Here's how the part is built. I have some questions about the finished solid (model axes, mm). A direction names the side the tool comes from. Coordinates: 2 decimals unless noted, no trailing zeros. Write each loop counter-clockwise with the first axis right and the second up, starting at its lowest first coordinate (ties: lowest second). Pieces come first, ordered by that corner, then holes. Notation, with made-up numbers: (-31, 13.25) -> (9, 13.25) arc R14 cw to (9, 35.25) -> close; hole circle Ø3 at (66.5, 67). An arc over 180 degrees is marked (long way). Use a Markdown table: item, result. Add a question column.
Item 1: If we mould it in two halves opening along X, with no side actions, what happens to faces 1 (the cylindrical face through (-59.462, -45.594, 6.261)), 2 (the cylindrical face through (184.06, 22.89, 117.82)), 3 (the cylindrical face through (-60.47, -46.367, 6.261))? For each: pulls with the +X half, pulls with the -X half, needs draft (parallel to the pull), parting line crosses it, or undercut.
Item 2: Imagine slicing it at A-A, the plane y = 0. Write out the boundary of the cut face in (x, z), and give its area (3 significant figures).
Item 3: Imagine slicing it at B-B, the plane y = -37. Write out the boundary of the cut face in (x, z).
Item 4: Will these pins go through, and if not, where does the flat tip stop? pin 1 Ø1.5 at (y, z) = (-53.5, 62) entering from -X; pin 2 Ø4 at (y, z) = (34.5, 58) entering from +X; pin 3 Ø3 at (x, y) = (107, -24) entering from +Z.
Item 5: If I drill on line 1 along Z through (x, y) = (179, 2); line 2 along Y through (x, z) = (186.25, 190.5); line 3 along Y through (x, z) = (-43, 60), over which ranges is the centre line in solid material (lowest first)? Write a range as from..to.
Item 6: On a 3-axis mill with a long thin cutter (end or side, diameter ignored), from which of +Z, -Z, +X, -X, +Y, -Y can I reach the whole of each face in a straight line? I mean faces 4 (the cylindrical face through (184.061, -28.699, 121.284)), 5 (the flat face through (190.5, -50, 134)). Say none if no direction works.
```python
from build123d import *

# Parameters (mm, degrees)
F0_R     = 76.2
F0_R_2   = 74.93
F1_DEPTH = 12.7
F2_R     = 76.2
F2_R_2   = 74.93
F3_ANGLE = 90
F4_DEPTH = 12.7


with BuildPart() as f1:
    # F0 (on Top) → F1 (new body)
    with BuildSketch(Plane.XY):
        Circle(F0_R)
        Circle(F0_R_2, mode=Mode.SUBTRACT)
    extrude(amount=F1_DEPTH)

    # F2 (on face) → F3 (revolve)
    with BuildSketch(Plane.XY.offset(12.7)):
        Circle(F2_R)
        Circle(F2_R_2, mode=Mode.SUBTRACT)
    revolve(axis=Axis((177.8, -2.9342612252, 12.7), (0, 1, 0)), revolution_arc=F3_ANGLE)

    # F4 (add): a face of the model
    f4_faces = [f1.faces().sort_by_distance(p)[0] for p in [
        (177.8, 0, 266.4844738531),
    ]]
    extrude(f4_faces, amount=F4_DEPTH)


solid = f1.part
```
Ans:
| question | item | result |
|---|---|---|
| 1 | face 1 | undercut |
| 1 | face 2 | needs draft |
| 1 | face 3 | parting line crosses it |
| 2 | outline | (-76.2, 0) -> (-74.93, 0) -> (-74.93, 12.7) arc R252.73 cw to (177.8, 265.43) -> (190.5, 265.43) -> (190.5, 266.7) -> (177.8, 266.7) arc R254 ccw to (-76.2, 12.7) -> close; (74.93, 0) -> (76.2, 0) -> (76.2, 12.7) arc R101.6 cw to (177.8, 114.3) -> (190.5, 114.3) -> (190.5, 115.57) -> (177.8, 115.57) arc R102.87 ccw to (74.93, 12.7) -> close |
| 2 | area | 774 mm^2 |
| 3 | outline | (-66.61, 0) -> (-65.16, 0) -> (-65.16, 12.7) arc R242.96 cw to (177.8, 255.66) -> (190.5, 255.66) -> (190.5, 257.11) -> (177.8, 257.11) arc R244.41 ccw to (-66.61, 12.7) -> close; (65.16, 0) -> (66.61, 0) -> (66.61, 12.7) arc R111.19 cw to (177.8, 123.89) -> (190.5, 123.89) -> (190.5, 125.34) -> (177.8, 125.34) arc R112.64 ccw to (65.16, 12.7) -> close |
| 4 | pin 1 | stops at x = -49.73 |
| 4 | pin 2 | stops at x = 79.15 |
| 4 | pin 3 | stops at z = 253.26 |
| 5 | line 1 | z = 114.33..115.6, 265.4..266.67 |
| 5 | line 2 | y = -76.2..-74.93, 74.93..76.2 |
| 5 | line 3 | y = -59.17..-57.53, 57.53..59.17 |
| 6 | face 4 | +X |
| 6 | face 5 | +Z, -Z, +X, +Y, -Y |
